```python
from build123d import *

# Parameters (mm, degrees)
F0_R     = 3
F0_R_2   = 1.75
F1_DEPTH = 15


with BuildPart() as f1:
    # F0 (on Right) → F1 (new body)
    with BuildSketch(Plane.YZ):
        with BuildLine():
            ThreePointArc((33.6642538877, 94.2964592226), (31.9768261624, 97.4851943073), (28.7658063512, 99.1298205687))
            add(Edge.make_bspline(
                [(28.7658063512, 99.1298205687), (19.203840359, 100.7513284104), (0.0799083746, 105.0635755317), (-19.0440236097, 100.7513284104), (-28.6059896019, 99.1298205687)],
                knots=[0.0624771081, 0.0624771081, 0.0624771081, 0.0624771081, 0.5, 0.9375228919, 0.9375228919, 0.9375228919, 0.9375228919], degree=3))
            ThreePointArc((-28.6059896019, 99.1298205687), (-31.8170094131, 97.4851943073), (-33.5044371384, 94.2964592226))
            add(Edge.make_bspline(
                [(-33.5044371384, 94.2964592226), (-35.6369863321, 82.6667901388), (-38.2031969186, 59.4074519711), (-35.6369863321, 36.1481138033), (-33.5044371384, 24.5184447195)],
                knots=[0.0534866237, 0.0534866237, 0.0534866237, 0.0534866237, 0.5, 0.9465133763, 0.9465133763, 0.9465133763, 0.9465133763], degree=3))
            ThreePointArc((-33.5044371384, 24.5184447195), (-31.8170094131, 21.3297096348), (-28.6059896019, 19.6850833734))
            add(Edge.make_bspline(
                [(-28.6059896019, 19.6850833734), (-19.0440236097, 18.0635755317), (0.0799083746, 13.7513284104), (19.203840359, 18.0635755317), (28.7658063512, 19.6850833734)],
                knots=[0.0624771081, 0.0624771081, 0.0624771081, 0.0624771081, 0.5, 0.9375228919, 0.9375228919, 0.9375228919, 0.9375228919], degree=3))
            ThreePointArc((28.7658063512, 19.6850833734), (31.9768261624, 21.3297096348), (33.6642538877, 24.5184447195))
            add(Edge.make_bspline(
                [(33.6642538877, 24.5184447195), (35.7968030814, 36.1481138033), (38.3630136679, 59.4074519711), (35.7968030814, 82.6667901388), (33.6642538877, 94.2964592226)],
                knots=[0.0534866237, 0.0534866237, 0.0534866237, 0.0534866237, 0.5, 0.9465133763, 0.9465133763, 0.9465133763, 0.9465133763], degree=3))
        make_face()
        with Locations((-28.8455340613, 24.9354520307)):
            Circle(F0_R, mode=Mode.SUBTRACT)
        with Locations((29.0053508105, 24.9354520307)):
            Circle(F0_R, mode=Mode.SUBTRACT)
        with Locations((-28.8455340613, 93.8794519114)):
            Circle(F0_R, mode=Mode.SUBTRACT)
        with Locations((29.0053508105, 93.8794519114)):
            Circle(F0_R, mode=Mode.SUBTRACT)
        with Locations((29.0053508105, 93.8794519114)):
            Circle(F0_R)
        with Locations((29.0053508105, 93.8794519114)):
            Circle(F0_R_2, mode=Mode.SUBTRACT)
        with Locations((-28.8455340613, 93.8794519114)):
            Circle(F0_R)
        with Locations((-28.8455340613, 93.8794519114)):
            Circle(F0_R_2, mode=Mode.SUBTRACT)
        with Locations((-28.8455340613, 24.9354520307)):
            Circle(F0_R)
        with Locations((-28.8455340613, 24.9354520307)):
            Circle(F0_R_2, mode=Mode.SUBTRACT)
        with Locations((29.0053508105, 24.9354520307)):
            Circle(F0_R)
        with Locations((29.0053508105, 24.9354520307)):
            Circle(F0_R_2, mode=Mode.SUBTRACT)
    extrude(amount=F1_DEPTH)


solid = f1.part
```
Source: CAD feature listing. Evaluate the final solid. Frame: model axes, mm. Round coordinates to 2 decimals unless told otherwise and drop trailing zeros.
1. Contact query for flat-ended pins moving along their axis: pin 1 (6 mm diameter, centred on x = 4, y = 16.5, fed in from +Z); pin 2 (1.5 mm diameter, centred on x = 7.5, z = 50, fed in from +Y). Output: stop coordinate, or through.
2. Section query A-A on x = 4. Give the number of separate pieces and of enclosed holes in the cut face, and give its area (3 significant figures).
3. Mould query, pull axis Z, two halves, no side actions, for faces 1 (the cylindrical face through (7.4, -30.23, 92.81)), 2 (the cylindrical face through (7.395, 31.94, 21.294)), 3 (the cylindrical face through (7.4, -31.8, 97.5)), 4 (the flat face through (0, 0, 60)). Classes: released by +Z, released by -Z, zero draft, split by the parting line, or undercut.
4. Ray query, L1, parallel to Z at x = 12.75, y = 29.5; L2, parallel to Y at x = 8.75, z = 59; L3, parallel to Y at x = 4, z = 34. Return the intervals inside material, ascending.
Answers below:
1. pin 1: stops at z = 101.77
1. pin 2: stops at y = 36.85
2. separate pieces: 1
2. enclosed holes: 4
2. area: 5,850 mm2
3. face 1: undercut
3. face 2: released by -Z
3. face 3: released by +Z
3. face 4: zero draft
4. L1: z = 19.86 to 23.26, 26.61 to 92.2, 95.56 to 98.96
4. L2: y = -36.92 to 37.08
4. L3: y = -35.05 to 35.21
